```python
from build123d import *

# Parameters (mm, degrees)
F0_R     = 31.75
F0_R_2   = 25.4
F1_DEPTH = 152.4
F3_DEPTH = 31.75
F4_R     = 6.35
F5_DEPTH = 31.75
F6_W     = 8.89
F6_H     = 25.4
F7_DEPTH = 38.1


with BuildPart() as f1:
    # F0 (on Top) → F1 (new body)
    with BuildSketch(Plane.XY):
        Circle(F0_R)
        Circle(F0_R_2, mode=Mode.SUBTRACT)
    extrude(amount=F1_DEPTH)

    # F2 (on Right) → F3 (cut, symmetric)
    with BuildSketch(Plane.YZ):
        Polygon((-31.75, 0), (31.75, 0), (31.75, 23.1121098759), align=None)
    extrude(amount=F3_DEPTH, both=True, mode=Mode.SUBTRACT)

    # F4 (on Front) → F5 (cut, symmetric)
    with BuildSketch(Plane.XZ):
        with Locations((0, 106.2535495254)):
            Circle(F4_R)
    extrude(amount=F5_DEPTH, both=True, mode=Mode.SUBTRACT)

    # F6 (on Front) → F7 (cut)
    with BuildSketch(Plane.XZ):
        Rectangle(F6_W, F6_H)
    extrude(amount=F7_DEPTH, mode=Mode.SUBTRACT)


solid = f1.part
```
Source: CAD feature listing. Evaluate the final solid. Frame: model axes, mm. A direction names the side the tool comes from. Round coordinates to 2 decimals unless told otherwise and drop trailing zeros. Loops run counter-clockwise (first coordinate to the right, second up) from the corner with the lowest first, then second, coordinate; pieces in that order, holes last. Notation, with made-up numbers: M 52,-28.5 L 109,-28.5 A29 cw 109,-0.5 Z; hole C -36,55 d4. An arc over 180 degrees is marked long. Use a Markdown table: item, result. Add a question column.
1. Line query: line 1 (X direction, y = 0, z = 90); line 2 (Z direction, x = 0, y = -28.75). Output: solid intervals per line, ascending.
2. Contact query for flat-ended pins moving along their axis: P1, Ø5, axis at y = 13, z = 45, coming from the +X side; P2, Ø5, axis at y = -30, z = 9, coming from the +X side; P3, Ø5, axis at y = -24, z = 18.5, coming from the +X side; P4, Ø14.5, axis at x = 0, z = 106.25, coming from the -Y side. Output: stop coordinate, or through.
3. Reachability of faces 1 (the flat face through (0, -28, 12.7)), 2 (the cylindrical face through (-4.68, -28.222, 110.545)) from +Z, -Z, +X, -X, +Y, -Y: full face, straight path, thin tool, end or side. Return the list, or none.
4. Mould query, pull axis X, two halves, no side actions, for faces 3 (the flat face through (4.445, -28, 6)), 4 (the cylindrical face through (-6.883, -30.995, 75.191)), 5 (the flat face through (-14.3, 21.3, 152.4)). Classes: pulls with the +X half, pulls with the -X half, needs draft (parallel to the pull), parting line crosses it, or undercut.
5. Section query C-C on x = 0. Return the cut outline in (y, z).
6. Section query B-B on y = -17. Return the cut outline in (x, z).
7. Section query A-A on x = -14.5. Return the cut outline in (y, z).
8. Section query D-D on z = 131.5. Return the cut outline in (x, y), then the cut area to 3 significant figures.
Reported:
| question | item | result |
|---|---|---|
| 1 | line 1 | x = -31.75 to -25.4, 25.4 to 31.75 |
| 1 | line 2 | z = 12.7 to 99.9, 112.6 to 152.4 |
| 2 | P1 | stops at x = 29.96 |
| 2 | P2 | stops at x = 15.87 |
| 2 | P3 | stops at x = 23.36 |
| 2 | P4 | stops at y = -31.75 |
| 3 | face 1 | -Z, +Y, -Y |
| 3 | face 2 | +Y, -Y |
| 4 | face 3 | undercut |
| 4 | face 4 | parting line crosses it |
| 4 | face 5 | needs draft |
| 5 | outline | M -31.75,12.7 L -25.4,12.7 L -25.4,99.9 L -31.75,99.9 Z; M -31.75,112.6 L -25.4,112.6 L -25.4,152.4 L -31.75,152.4 Z; M 25.4,20.8 L 31.75,23.11 L 31.75,99.9 L 25.4,99.9 Z; M 25.4,112.6 L 31.75,112.6 L 31.75,152.4 L 25.4,152.4 Z |
| 6 | outline | M -26.82,5.37 L -18.87,5.37 L -18.87,152.4 L -26.82,152.4 Z; M 18.87,5.37 L 26.82,5.37 L 26.82,152.4 L 18.87,152.4 Z |
| 7 | outline | M -28.25,1.28 L -20.85,3.97 L -20.85,152.4 L -28.25,152.4 Z; M 20.85,19.15 L 28.25,21.84 L 28.25,152.4 L 20.85,152.4 Z |
| 8 | outline | C 0,0 d63.5; hole C 0,0 d50.8 |
| 8 | area | 1,140 mm² |
